Could you check a few things on this drawing? It's one solid part, dimensions in mm from its lowest x, y, z. A direction names the side the tool comes from. Round coordinates to 2 decimals unless told otherwise and drop trailing zeros. Loops run counter-clockwise (first coordinate to the right, second up) from the corner with the lowest first, then second, coordinate; pieces in that order, holes last. Notation, with made-up numbers: (45.25, 53) -> (50.25, 53) arc R22 ccw to (50.25, 92) -> close; hole circle Ø10 at (-10, 50.25). An arc over 180 degrees is marked (long way). Use one line per item in the form item = value. Start each with the question number.
Item 1: If we section it at C-C (x = 11.25): Write out the boundary of the cut face in (y, z), then the cut area to 3 significant figures.
Item 2: If we section it at B-B (z = 3): Write out the boundary of the cut face in (x, y), then the cut area to 3 significant figures.
Item 3: If I drill on L1, parallel to X at y = 0.75, z = 15; L2, parallel to X at y = 1.15, z = 3; L3, parallel to X at y = 1, z = 5, over which ranges is the centre line in solid material (lowest first)? Write a range as [from, to].
Item 4: Thinking about a two-plate mould opening in X: for the marked faces 4, 5 and 6, which applies, released by +X, released by -X, zero draft, split by the parting line, or undercut?
Item 5: If we section it at D-D (z = 17): Write out the boundary of the cut face in (x, y).
Item 6: For the marked faces 1, 2 and 3, which set-ups out of +Z, -Z, +X, -X, +Y, -Y let a thin tool reach every point of the face, with its end or its side?
Item 7: I'm going to push flat-ended pins straight in: pin 1 Ø0.6 at (y, z) = (1, 19.5) entering from -X; pin 2 Ø1.5 at (x, y) = (20, 1) entering from +Z; pin 3 Ø1 at (y, z) = (2, 18.5) entering from +X. Where does each tip first touch, or does it pass through?
Item 8: If we section it at A-A (y = 0.45): Write out the boundary of the cut face in (x, z), then the cut area to 3 significant figures.
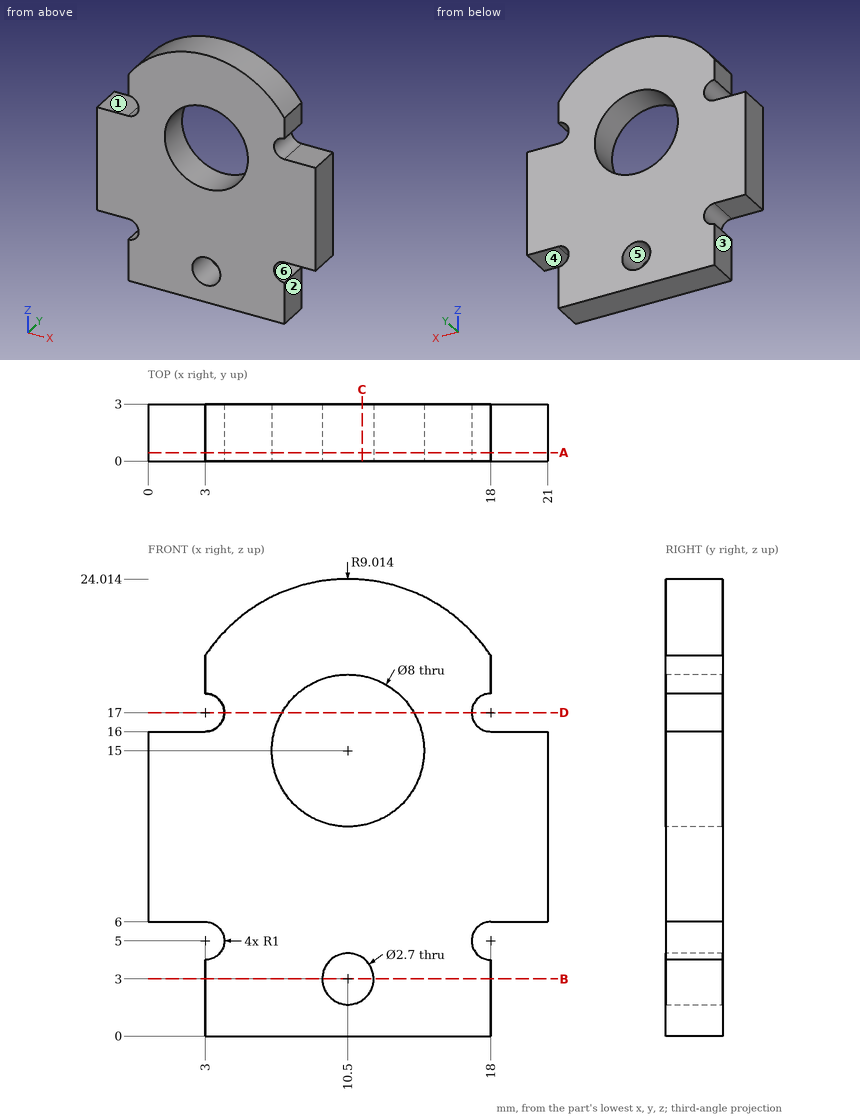
Values found:
q1.outline = (0, 0) -> (3, 0) -> (3, 1.88) -> (0, 1.88) -> close; (0, 4.12) -> (3, 4.12) -> (3, 11.07) -> (0, 11.07) -> close; (0, 18.93) -> (3, 18.93) -> (3, 23.98) -> (0, 23.98) -> close
q1.area = 41.6 mm2
q2.outline = (3, 0) -> (9.15, 0) -> (9.15, 3) -> (3, 3) -> close; (11.85, 0) -> (18, 0) -> (18, 3) -> (11.85, 3) -> close
q2.area = 36.9 mm2
q3.L1 = [0, 6.5], [14.5, 21]
q3.L2 = [3, 9.15], [11.85, 18]
q3.L3 = [4, 17]
q4.face_4 = zero draft
q4.face_5 = undercut
q4.face_6 = released by +X
q5.outline = (4, 0) -> (7.04, 0) -> (7.04, 3) -> (4, 3) -> close; (13.96, 0) -> (17, 0) -> (17, 3) -> (13.96, 3) -> close
q6.face_1 = +Z, -X, +Y, -Y
q6.face_2 = -Z, +X, +Y, -Y
q6.face_3 = -Z, -X, +Y, -Y
q7.pin_1 = 3
q7.pin_2 = 16
q7.pin_3 = 18
q8.outline = (0, 6) -> (3, 6) arc R1 cw to (3, 4) -> (3, 0) -> (18, 0) -> (18, 4) arc R1 cw to (18, 6) -> (21, 6) -> (21, 16) -> (18, 16) arc R1 cw to (18, 18) -> (18, 20) arc R9.01 ccw to (3, 20) -> (3, 18) arc R1 cw to (3, 16) -> (0, 16) -> close; hole circle Ø8 at (10.5, 15); hole circle Ø2.7 at (10.5, 3)
q8.area = 340 mm2
